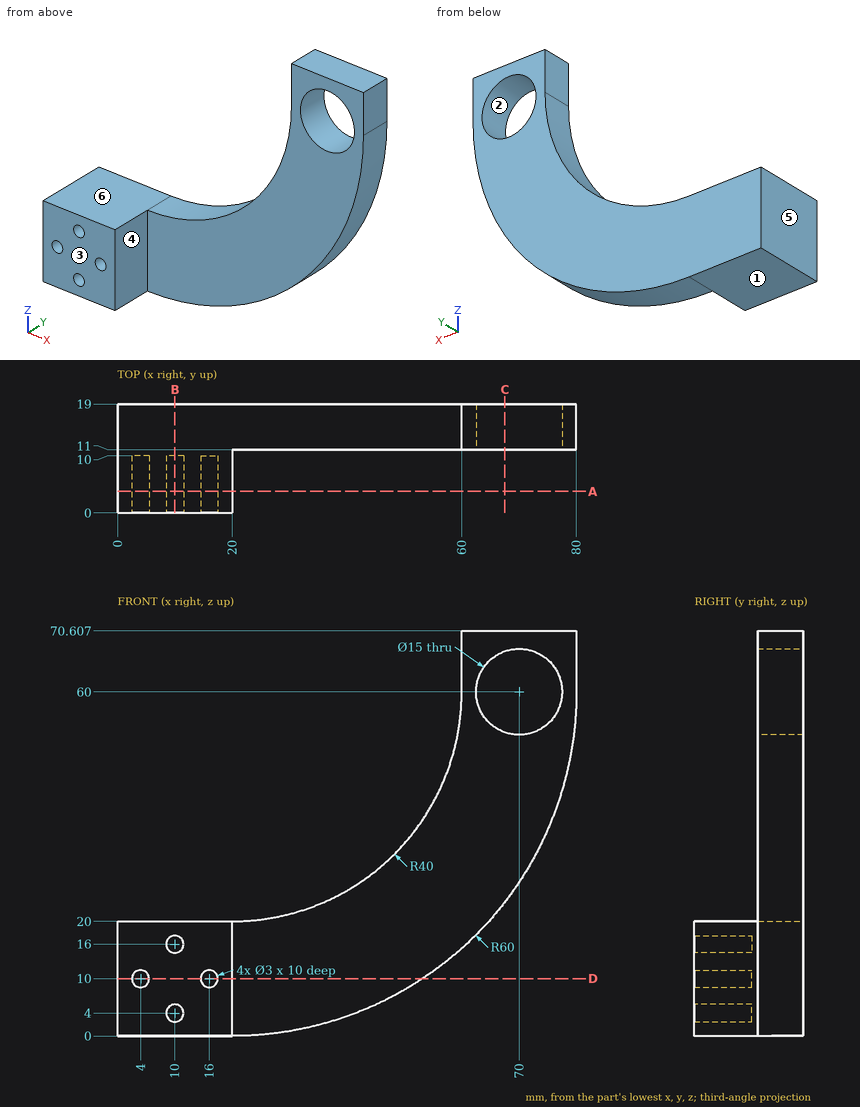
Study the drawing (mm; zero at the part's minimum x, y, z) and answer. A direction names the side the tool comes from. Coordinates: 2 decimals unless noted, no trailing zeros. Write each loop counter-clockwise with the first axis right and the second up, starting at its lowest first coordinate (ties: lowest second). Pieces come first, ordered by that corner, then holes. Notation, with made-up numbers: (30.25, -32.5) - (69.25, -32.5) arc R33 cw to (69.25, 3.5) - close; hole circle Ø9 at (39, 15.5). An arc over 180 degrees is marked (long way). Answer as a JSON object with one key per item and string values. Group by question number.
1. Consider L1, parallel to X at y = 6, z = 10; L2, parallel to Z at x = 16, y = 2. Determine where each line is inside the solid, lowest interval first. Write a range as [from, to].
2. The mould has two halves that part along Z. Classify the marked faces 1, 2 and 3: +Z half, -Z half, draft (parallel to the pull), parting line (faces both ways), or undercut.
3. Which of the six approach directions +Z, -Z, +X, -X, +Y, -Y give full straight-line access (tool end or side, diameter ignored) to the marked faces 4, 5 and 6?
4. A cutting plane is placed at B-B (x = 10). Determine the outline of the cut face in (y, z), plus the area to 3 significant figures.
5. A cutting plane is placed at A-A (y = 3.75). Determine the outline of the cut face in (x, z), plus the area to 3 significant figures.
6. A cutting plane is placed at D-D (z = 10). Determine the outline of the cut face in (x, y), plus the area to 3 significant figures.
7. A cutting plane is placed at C-C (x = 67.5). Determine the outline of the cut face in (y, z).
8. Each of these flat-tipped pins is pushed along its axis until it touches: P1, Ø2.5, axis at x = 16, z = 10, coming from the -Y side; P2, Ø2.5, axis at x = 4, z = 9.5, coming from the -Y side; P3, Ø4, axis at y = 15.5, z = 67, coming from the -X side; P4, Ø1, axis at x = 9.5, z = 22, coming from the +Y side. Where does it stop, or does it pass through?
Worked out:
{
 "1": {"L1": "x = [0, 2.5], [5.5, 14.5], [17.5, 20]", "L2": "z = [0, 8.5], [11.5, 20]"},
 "2": {"face 1": "-Z half", "face 2": "undercut", "face 3": "draft"},
 "3": {"face 4": "+Z, -Z, +X, -Y", "face 5": "+Z, -Z, -X, +Y, -Y", "face 6": "+Z, -X, +Y, -Y"},
 "4": {"outline": "(0, 0) - (19, 0) - (19, 20) - (0, 20) - (0, 17.5) - (10, 17.5) - (10, 14.5) - (0, 14.5) - (0, 5.5) - (10, 5.5) - (10, 2.5) - (0, 2.5) - close", "area": "320 mm²"},
 "5": {"outline": "(0, 0) - (20, 0) - (20, 20) - (0, 20) - close; hole circle Ø3 at (4, 10); hole circle Ø3 at (10, 4); hole circle Ø3 at (10, 16); hole circle Ø3 at (16, 10)", "area": "372 mm²"},
 "6": {"outline": "(0, 0) - (2.5, 0) - (2.5, 10) - (5.5, 10) - (5.5, 0) - (14.5, 0) - (14.5, 10) - (17.5, 10) - (17.5, 0) - (20, 0) - (20, 11) - (53.17, 11) - (53.17, 19) - (0, 19) - close", "area": "585 mm²"},
 "7": {"outline": "(11, 23.34) - (19, 23.34) - (19, 52.93) - (11, 52.93) - close; (11, 67.07) - (19, 67.07) - (19, 70.61) - (11, 70.61) - close"},
 "8": {"P1": "stops at y = 10", "P2": "stops at y = 0", "P3": "stops at x = 60", "P4": "passes through"}
}
